Autodesk Inventor part; units mm, degrees
ref_plane "Work Plane1" through (0, 8, 0) normal (0, 1, 0) x (1, 0, 0)
ref_plane "YZ Plane" through (0, 0, 0) normal (1, 0, 0) x (0, 1, 0)
ref_plane "XZ Plane" through (0, 0, 0) normal (0, 1, 0) x (-1, 0, 0)
sketch "Sketch1" plane through (0, 0, 0) normal (0, 1, 0) x (-1, 0, 0)
  arc A0 (31.569, 13.7227) -> (30.069, 12.2227) centre (31.569, 12.2227) ccw
  line L0 (31.569, 13.7227) -> (34.069, 13.7227)
  line L1 (34.069, 13.7227) -> (34.069, 18.9227)
  line L2 (32.069, 20.9227) -> (2.569, 20.9227)
  line L3 (34.069, -13.2773) -> (31.569, -13.2773)
  arc A1 (30.069, -11.7773) -> (31.569, -13.2773) centre (31.569, -11.7773) ccw
  arc A2 (34.069, 18.9227) -> (32.069, 20.9227) centre (32.069, 18.9227) ccw
  arc A3 (34.0195, 22.4149) -> (32.069, 23.9727) centre (32.069, 21.9727) ccw
  line L4 (32.069, 23.9727) -> (-23.931, 23.9727)
  arc A4 (-23.931, 23.9727) -> (-25.931, 21.9727) centre (-23.931, 21.9727) ccw
  line L5 (-25.931, 21.9727) -> (-25.931, -21.0273)
  arc A5 (-25.931, -21.0273) -> (-23.931, -23.0273) centre (-23.931, -21.0273) ccw
  line L6 (-23.931, -23.0273) -> (32.069, -23.0273)
  arc A6 (32.069, -23.0273) -> (33.899, -21.8341) centre (32.069, -21.0273) ccw
  arc A7 (32.069, -20.2773) -> (34.069, -18.2773) centre (32.069, -18.2773) ccw
  line L7 (32.069, -20.2773) -> (0.569, -20.2773)
  line L8 (34.069, -13.2773) -> (34.069, 13.7227)
  line L9 (0.569, -22.2773) -> (0.569, 18.9227)
  line L10 (30.069, -11.7773) -> (30.069, 12.2227)
  line L11 (34.069, -18.2773) -> (34.069, -13.2773)
  line L12 (2.569, 22.9227) -> (32.069, 22.9227)
  line L13 (0.569, -22.2773) -> (32.069, -22.2773)
  arc A8 (32.069, -22.2773) -> (36.069, -18.2773) centre (32.069, -18.2773) ccw
  line L14 (36.069, -18.2773) -> (36.069, 18.9227)
  arc A9 (2.569, 20.9227) -> (0.569, 18.9227) centre (2.569, 18.9227) ccw
  line L15 (-1.431, 14.4227) -> (-1.431, 18.9227)
  arc A10 (2.569, 22.9227) -> (-1.431, 18.9227) centre (2.569, 18.9227) ccw
  arc A11 (36.069, 18.9227) -> (32.069, 22.9227) centre (32.069, 18.9227) ccw
  line L16 (-1.431, 14.4227) -> (0.569, 14.4227)
  point P0 (0.569, 20.9227)
  dimension "d8" = 2
  dimension "d9" = 2
  dimension "d66" = 2
  dimension "d67" = 2
  dimension "d68" = 4.5
  dimension "d69" = 4
extrude "Extrusion3" add sketch "Sketch1" against normal blind 2 contours L0 L8 L3 A1 L10 A0 | A0 L10 A1 L3 L11 A7 L7 L9 A9 L2 A2 L1 L0 | L1 A2 L2 A9 L9 L16 L15 A10 L12 A11 L14 A8 L13 L7 A7 L11 L8
ref_plane "Work Plane1" through (0, 8, 0) normal (0, 1, 0) x (1, 0, 0)
extrude "Extrusion4" add sketch "Sketch1" along normal blind 8 contours L1 A2 L2 A9 L9 L16 L15 A10 L12 A11 L14 A8 L13 L7 A7 L11 L8
sketch "Sketch2" plane through (0, 8, 0) normal (0, 1, 0) x (1, 0, 0)
  line L0 (23.931, 23.0273) -> (-32.069, 23.0273)
  arc A0 (-32.069, 23.0273) -> (-33.899, 21.8341) centre (-32.069, 21.0273) ccw
  line L1 (-32.069, -23.9727) -> (23.931, -23.9727)
  arc A1 (-34.0195, -22.4149) -> (-32.069, -23.9727) centre (-32.069, -21.9727) ccw
  arc A2 (-32.069, 23.0273) -> (-34.069, 21.0273) centre (-32.069, 21.0273) ccw
  arc A3 (-34.069, -21.9727) -> (-32.069, -23.9727) centre (-32.069, -21.9727) ccw
  line L2 (-34.069, 18.2773) -> (-34.069, 13.2773)
  line L3 (-34.069, 13.2773) -> (-34.069, -13.7227)
  line L4 (-34.069, -13.7227) -> (-34.069, -18.9227)
  line L5 (-34.069, -21.9727) -> (-34.069, 21.0273)
  arc A4 (-32.069, 25.0273) -> (-36.069, 21.0273) centre (-32.069, 21.0273) ccw
  line L6 (-0.569, 25.0273) -> (-32.069, 25.0273)
  line L7 (-0.569, -25.9727) -> (-32.069, -25.9727)
  line L8 (-0.569, -23.9727) -> (-0.569, -25.9727)
  line L9 (-0.569, 20.2773) -> (-0.569, 25.0273)
  line L10 (-0.569, 22.2773) -> (-0.569, 22.2773)
  line L11 (-32.069, 23.0273) -> (-0.569, 23.0273)
  line L12 (-32.069, -23.9727) -> (-0.569, -23.9727)
  line L13 (-32.069, -20.9227) -> (-2.569, -20.9227)
  line L14 (-0.569, -14.4227) -> (-0.569, 20.2773)
  line L15 (-0.569, 20.2773) -> (-32.069, 20.2773)
  arc A5 (-32.069, 20.2773) -> (-34.069, 18.2773) centre (-32.069, 18.2773) ccw
  line L16 (-34.069, 18.2773) -> (-34.069, -18.9227)
  arc A6 (-34.069, -18.9227) -> (-32.069, -20.9227) centre (-32.069, -18.9227) ccw
  line L17 (-32.069, 22.2773) -> (-0.569, 22.2773)
  line L18 (-0.569, 22.2773) -> (-0.569, 22.2773)
  arc A7 (-2.569, -20.9227) -> (-0.569, -18.9227) centre (-2.569, -18.9227) ccw
  line L19 (-0.569, -18.9227) -> (-0.569, -14.4227)
  line L20 (-0.569, -23.9727) -> (-0.569, -18.9227)
  line L21 (-36.069, 21.0273) -> (-36.069, -21.9727)
  arc A8 (-36.069, -21.9727) -> (-32.069, -25.9727) centre (-32.069, -21.9727) ccw
  point P0 (0, 0)
  point P1 (-32.069, 25.0273)
  dimension "d19" = 2
  dimension "d20" = 2
  dimension "d21" = 31.5
  dimension "d22" = 31.5
  dimension "d23" = 31.5
extrude "Extrusion7" add sketch "Sketch2" against normal blind 2 contours L9 L15 A5 L5 A2 A0 L0 | L0 A0 A2 L5 L2 L3 L4 A3 A1 L1 L8 L7 A8 L21 A4 L6 L9 | L20 L1 A1 A3 L5 A6 L13 A7
extrude "Extrusion8" add sketch "Sketch2" along normal blind 15 contours L0 A0 A2 L5 L2 L3 L4 A3 A1 L1 L8 L7 A8 L21 A4 L6 L9
sketch "Sketch5" plane through (0, 23, 0) normal (0, 1, 0) x (1, 0, 0)
  circle A0 centre (-17.319, 30.0273) radius 5
  circle A1 centre (-17.319, 30.0273) radius 3
  arc A2 (-12.4777, 28.7773) -> (-9.573, 25.0273) centre (-9.573, 28.0273) ccw
  arc A3 (-25.0649, 25.0273) -> (-22.1602, 28.7773) centre (-25.0649, 28.0273) ccw
  line L0 (-0.569, 23.0273) -> (-0.569, 25.0273)
  circle A4 centre (-6.0917, -30.9727) radius 5
  circle A5 centre (-6.0917, -30.9727) radius 3
  arc A6 (-10.305, -28.2804) -> (-11.569, -25.9727) centre (-11.569, -27.4727) ccw
  arc A7 (-0.6145, -25.9727) -> (-1.8785, -28.2804) centre (-0.6145, -27.4727) ccw
  circle A8 centre (-26.5917, -30.9727) radius 5
  circle A9 centre (-26.5917, -30.9727) radius 3
  arc A10 (-30.805, -28.2804) -> (-32.069, -25.9727) centre (-32.069, -27.4727) ccw
  arc A11 (-21.1145, -25.9727) -> (-22.3785, -28.2804) centre (-21.1145, -27.4727) ccw
  line L1 (-0.569, -25.9727) -> (-0.569, -23.9727)
  line L2 (-0.569, 25.0273) -> (-32.069, 25.0273)
  line L3 (-32.069, -25.9727) -> (-0.569, -25.9727)
  point P0 (0, 0)
  point P1 (1.0185, -24.3852)
  point P2 (-26.5917, -25.9727)
  point P3 (-6.0917, -25.9727)
  point P4 (-17.319, 25.0273)
  dimension "d34" = 10
  dimension "d35" = 6
  dimension "d38" = 3
  dimension "d39" = 3
  dimension "d40" = 10
  dimension "d41" = 6
  dimension "d42" = 3
  dimension "d43" = 3
  dimension "d44" = 10
  dimension "d45" = 6
  dimension "d46" = 3
  dimension "d47" = 3
  dimension "d49" = 20.5
extrude "Extrusion10" add sketch "Sketch5" against normal blind 2.5
sketch "Sketch6" plane through (0, -2, 0) normal (0, -1, 0) x (1, 0, 0)
  line L0 (-0.569, -22.2773) -> (-0.569, 14.4227)
  line L1 (-2.569, 22.9227) -> (-32.069, 22.9227)
  arc A0 (-32.069, 22.9227) -> (-36.069, 18.9227) centre (-32.069, 18.9227) ccw
  line L2 (-36.069, 18.9227) -> (-36.069, -18.2773)
  arc A1 (-36.069, -18.2773) -> (-32.069, -22.2773) centre (-32.069, -18.2773) ccw
  line L3 (-32.069, -22.2773) -> (-0.569, -22.2773)
  line L4 (-30.069, 18.9227) -> (-6.569, 18.9227)
  line L5 (-4.569, 16.9227) -> (-4.569, -16.2773)
  line L6 (-6.569, -18.2773) -> (-30.069, -18.2773)
  line L7 (-32.069, -16.2773) -> (-32.069, 16.9227)
  arc A2 (-6.569, -18.2773) -> (-4.569, -16.2773) centre (-6.569, -16.2773) ccw
  arc A3 (-32.069, -16.2773) -> (-30.069, -18.2773) centre (-30.069, -16.2773) ccw
  arc A4 (-30.069, 18.9227) -> (-32.069, 16.9227) centre (-30.069, 16.9227) ccw
  arc A5 (-4.569, 16.9227) -> (-6.569, 18.9227) centre (-6.569, 16.9227) ccw
  line L8 (-0.569, 14.4227) -> (1.431, 14.4227)
  line L9 (1.431, 14.4227) -> (1.431, 18.9227)
  arc A6 (1.431, 18.9227) -> (-2.569, 22.9227) centre (-2.569, 18.9227) ccw
  point P0 (0, 0)
  point P1 (-4.569, 18.9227)
  point P2 (-4.569, -18.2773)
  dimension "d52" = 4
  dimension "d53" = 37.2
  dimension "d54" = 27.5
  dimension "d55" = 4
  dimension "d56" = 2
extrude "Extrusion11" cut sketch "Sketch6" against normal blind 2 contours L4 A5 L5 A2 L6 A3 L7 A4
sketch "Sketch7" plane through (-36.069, -2, -18.2773) normal (-1, 0, 0) x (0, 0, 1)
  line L0 (2.75, 25) -> (34.75, 25)
  line L1 (34.75, 25) -> (34.75, 17)
  line L2 (32.75, 15) -> (4.75, 15)
  line L3 (2.75, 17) -> (2.75, 25)
  arc A0 (2.75, 17) -> (4.75, 15) centre (4.75, 17) ccw
  arc A1 (32.75, 15) -> (34.75, 17) centre (32.75, 17) ccw
  point P0 (18.2773, 2)
  point P1 (40.25, 25)
  point P2 (-2.75, 25)
  point P3 (34.75, 21)
  point P4 (40.25, 8)
  dimension "d59" = 2
  dimension "d61" = 32
  dimension "d62" = 43
extrude "Extrusion12" cut sketch "Sketch7" against normal blind 6
sketch "Sketch8" plane through (0, 8, 0) normal (0, 1, 0) x (1, 0, 0)
  line L0 (-0.569, -14.4227) -> (-0.569, -18.9227)
  line L1 (1.431, -14.4227) -> (-0.569, -14.4227)
  line L2 (1.431, -18.9227) -> (1.431, -14.4227)
  arc A0 (-0.569, -22.3868) -> (1.431, -18.9227) centre (-2.569, -18.9227) ccw
  line L3 (-0.569, -23.9727) -> (-0.569, -18.9227)
  point P0 (0, 0)
extrude "Extrusion13" cut sketch "Sketch8" against normal blind 6
properties part number "CO-1-01-motorControllersMount"
Verification items for the finished model (mm, model axes). A direction names the side the tool comes from. Give positions to 0.01 mm unless a question says otherwise; leave off trailing zeros. Write each loop counter-clockwise with the first axis right and the second up, starting at its lowest first coordinate (ties: lowest second). Pieces come first, ordered by that corner, then holes.
(1) Cross-section at B-B (z = 2). Enter the section's corners in (x, y).
(2) Cross-section at A-A (y = 16.25). Enter the section's corners in (x, z), plus the area to 3 significant figures.
(3) Cross-section at C-C (y = 3.5). Enter the section's corners in (x, z), plus the area to 3 significant figures.
(4) Mould release check, pull along X, two halves, no side actions. Record for faces 4 (the face through (-4.479, 21.768, 28.443)), 5 (the face through (-35, 2, -21)), 6 (the face through (-22.4, 21.8, 26.7)), 7 (the face through (-35, 13, 1)): +X half, -X half, draft (parallel to the pull), parting line (faces both ways), or undercut.
(5) Cross-section at D-D (z = 29). Enter the section's corners in (x, y), plus the area to 3 significant figures.
(6) Access from +Z, -Z, +X, -X, +Y, -Y to the whole of each face (thin tool, end or side, straight path). Record for faces 1 (the face through (-0.239, 1.055, 22.174)), 2 (the face through (-18, -1, 18.923)), 3 (the face through (-17, 8, 23)).
(7) Material ranges on line 1 (Z direction, x = -20.5, y = 6.5); line 2 (Z direction, x = -2.5, y = 17.25); line 3 (X direction, y = -1, z = 7.5), recorded low to high.
(8) Gauge pin test, flat ends, axial feed: pin 1 (1.5 mm diameter, centred on x = -9, z = -18, fed in from +Y); pin 2 (1.6 mm diameter, centred on x = 0.5, z = 19.5, fed in from +Y); pin 3 (6.5 mm diameter, centred on x = -21, y = 3, fed in from +Z). Record the tip position at first contact, or that the pin passes through.
Worked out:
1. outline: (-36.07, -2) - (-32.07, -2) - (-32.07, 0) - (-34.07, 0) - (-34.07, 13) - (-36.07, 13) - close; (-4.57, -2) - (-0.57, -2) - (-0.57, 0) - (-4.57, 0) - close
2. outline: (-36.07, -21.03) arc R4 ccw to (-32.07, -25.03) - (-0.57, -25.03) - (-0.57, -23.03) - (-32.07, -23.03) arc R2 cw to (-33.9, -21.83) arc R2 cw to (-34.07, -21.03) - (-34.07, -15.53) - (-36.07, -15.53) - close; (-36.07, 16.47) - (-34.07, 16.47) - (-34.07, 21.97) arc R2 cw to (-34.02, 22.41) arc R2 cw to (-32.07, 23.97) - (-0.57, 23.97) - (-0.57, 25.97) - (-32.07, 25.97) arc R4 ccw to (-36.07, 21.97) - close
2. area: 167 mm2
3. outline: (-36.07, -18.28) arc R4 ccw to (-32.07, -22.28) - (-0.57, -22.28) - (-0.57, -20.28) - (-32.07, -20.28) arc R2 cw to (-34.07, -18.28) - (-34.07, 18.92) arc R2 cw to (-32.07, 20.92) - (-2.57, 20.92) arc R2 cw to (-0.57, 18.92) - (-0.57, 22.39) arc R4 ccw to (-2.57, 22.92) - (-32.07, 22.92) arc R4 ccw to (-36.07, 18.92) - close
3. area: 220 mm2
4. face 4: undercut
4. face 5: -X half
4. face 6: undercut
4. face 7: draft
5. outline: (-31.19, 20.5) - (-28.85, 20.5) - (-28.85, 23) - (-31.19, 23) - close; (-24.33, 20.5) - (-22, 20.5) - (-22, 23) - (-24.33, 23) - close; (-10.69, 20.5) - (-8.35, 20.5) - (-8.35, 23) - (-10.69, 23) - close; (-3.83, 20.5) - (-1.5, 20.5) - (-1.5, 23) - (-3.83, 23) - close
5. area: 23.3 mm2
6. face 1: +Z, +X, -Y
6. face 2: +Y, -Y
6. face 3: +X, +Y
7. line 1: z = -25.03 to -20.28, 20.92 to 25.97
7. line 2: z = -25.03 to -23.03, 23.97 to 25.97
7. line 3: x = -36.07 to -32.07, -4.57 to -0.57
8. pin 1: stops at y = 0
8. pin 2: stops at y = 2
8. pin 3: stops at z = 25.97
